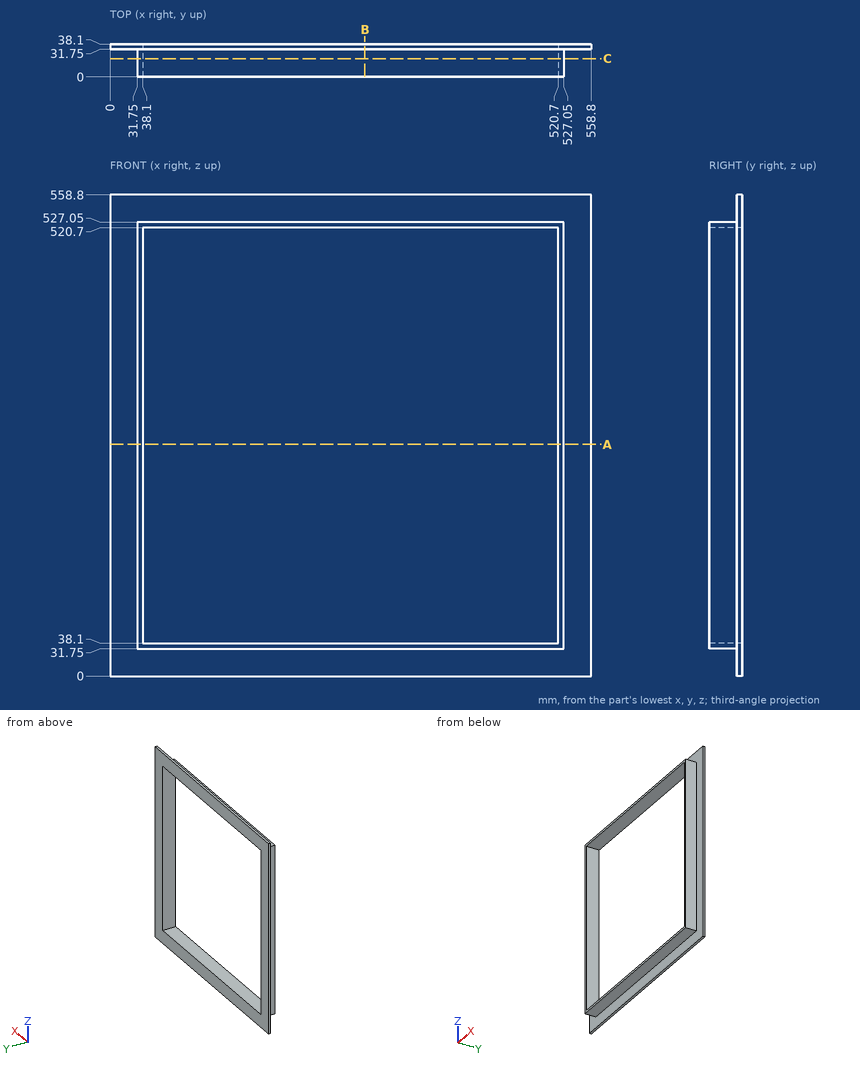
Print and shaded views of the part. All mm, measured from the part's lowest x, y and z. Give positions to 0.01 mm unless a question says otherwise; leave off trailing zeros. Write each loop counter-clockwise with the first axis right and the second up, starting at its lowest first coordinate (ties: lowest second). Pieces come first, ordered by that corner, then holes. Notation, with made-up numbers: (-35, 31) - (-16, 31) arc R17 cw to (-16, 44) - close; hole circle Ø8 at (80.25, 3). An arc over 180 degrees is marked (long way). One line per question, with ' | ' between items. Start each with the question number.
(1) Wall check: line 1 along X through (y, z) = (35.5, 206.5); line 2 along Z through (x, y) = (467.5, 12). Give the ranges that are in metal, low to high. Write a range as from..to.
(2) Slice it at B-B on x = 296. Write the cut outline in (y, z), plus the area to 3 significant figures.
(3) Pin check, flat tips, straight feed: P1, Ø11.5, axis at y = 15, z = 228, coming from the -X side; P2, Ø1, axis at y = 13.5, z = 295.5, coming from the +X side; P3, Ø9.5, axis at x = 374, y = 22, coming from the +Z side. Stop position of each tip, or through.
(4) Slice it at C-C on y = 21. Write the cut outline in (x, z), plus the area to 3 significant figures.
(5) Slice it at A-A on z = 269. Write the cut outline in (x, y), plus the area to 3 significant figures.
Results below:
1) line 1: 0..38.1, 520.7..558.8 | line 2: 31.75..38.1, 520.7..527.05
2) outline: (0, 31.75) - (31.75, 31.75) - (31.75, 0) - (38.1, 0) - (38.1, 38.1) - (0, 38.1) - close; (0, 520.7) - (38.1, 520.7) - (38.1, 558.8) - (31.75, 558.8) - (31.75, 527.05) - (0, 527.05) - close | area: 887 mm^2
3) P1: x = 31.75 | P2: x = 527.05 | P3: z = 527.05
4) outline: (31.75, 31.75) - (527.05, 31.75) - (527.05, 527.05) - (31.75, 527.05) - close; hole (38.1, 38.1) - (520.7, 38.1) - (520.7, 520.7) - (38.1, 520.7) - close | area: 12,400 mm^2
5) outline: (0, 31.75) - (31.75, 31.75) - (31.75, 0) - (38.1, 0) - (38.1, 38.1) - (0, 38.1) - close; (520.7, 0) - (527.05, 0) - (527.05, 31.75) - (558.8, 31.75) - (558.8, 38.1) - (520.7, 38.1) - close | area: 887 mm^2
